Read the model definition and answer for the solid it produces. Units are mm, in the model's axes. Coordinates: 2 decimals unless noted, no trailing zeros. Loops run counter-clockwise (first coordinate to the right, second up) from the corner with the lowest first, then second, coordinate; pieces in that order, holes last. Notation, with made-up numbers: (11, -15.75) -> (56, -15.75) arc R16 ccw to (56, -7.75) -> close; hole circle Ø3 at (-11.75, 23.5). An arc over 180 degrees is marked (long way). Answer as a JSON object with one key per item and string values. Group by question number.
Q1. The part is cut by section A-A on x = -90. Write down the section's boundary in (y, z).
Q2. This flat-tipped pin is pushed along its axis until it touches: P1, Ø6.5, axis at x = -90, y = -90, coming from the -Z side. Where does it stop, or does it pass through?
Q3. The part is cut by section C-C on x = 45. Write down the section's boundary in (y, z).
Q4. Straight lines are drawn through the part: line 1 along Y through (x, z) = (90, 2.5); line 2 along Y through (x, z) = (-45, 2.05). For each, find the intervals that lie inside material, in ascending order. Write a range as [from, to].
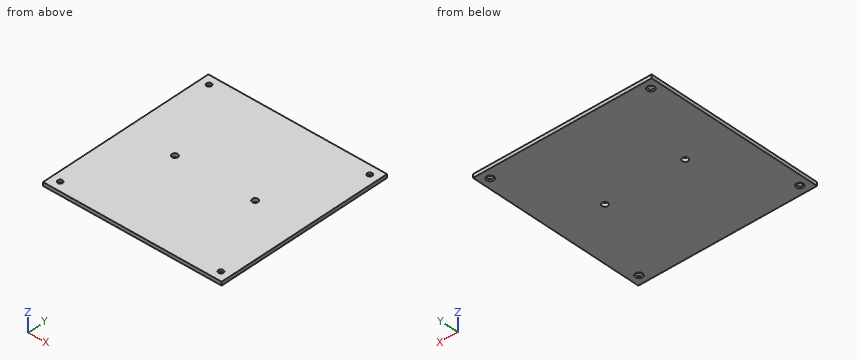
from build123d import *

# Parameters (mm, degrees)
F0_W           = 200
F0_H           = 200
F1_DEPTH       = 4
F2_D           = 5.5
F2_CSINK_D     = 8
F2_CSINK_ANGLE = 90
F3_D           = 6.6


with BuildPart() as f1:
    # F0 (on Top) → F1 (new body)
    with BuildSketch(Plane.XY):
        Rectangle(F0_W, F0_H)
    extrude(amount=F1_DEPTH)

    # F2 (through all)
    with Locations(Plane(origin=(0, 0, 0), x_dir=(1, 0, 0), z_dir=(0, 0, -1))):
        with Locations((-90, 90), (90, 90), (90, -90), (-90, -90)):
            CounterSinkHole(F2_D / 2, F2_CSINK_D / 2, counter_sink_angle=F2_CSINK_ANGLE)

    # F3 (through all)
    with Locations(Plane(origin=(0, 0, 0), x_dir=(1, 0, 0), z_dir=(0, 0, -1))):
        with Locations((45, 0), (-45, 0)):
            Hole(F3_D / 2)


solid = f1.part
Final values:
{
 "1": {"outline": "(-100, 0) -> (-94, 0) -> (-92.75, 1.25) -> (-92.75, 4) -> (-100, 4) -> close; (-87.25, 1.25) -> (-86, 0) -> (86, 0) -> (87.25, 1.25) -> (87.25, 4) -> (-87.25, 4) -> close; (92.75, 1.25) -> (94, 0) -> (100, 0) -> (100, 4) -> (92.75, 4) -> close"},
 "2": {"P1": "stops at z = 0.75"},
 "3": {"outline": "(-100, 0) -> (-3.3, 0) -> (-3.3, 4) -> (-100, 4) -> close; (3.3, 0) -> (100, 0) -> (100, 4) -> (3.3, 4) -> close"},
 "4": {"line 1": "y = [-100, -92.75], [-87.25, 87.25], [92.75, 100]", "line 2": "y = [-100, -3.3], [3.3, 100]"}
}
